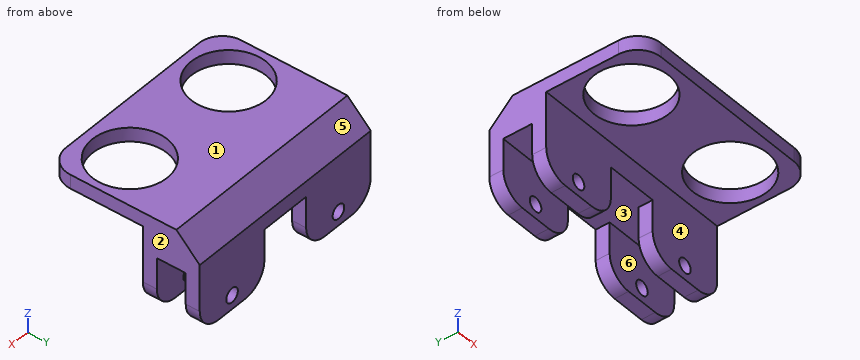
```python
from build123d import *

# Parameters (mm, degrees)
SKETCH1_R           = 8
BOSS_EXTRUDE1_DEPTH = 3
SKETCH2_W           = 17
SKETCH2_H           = 3
BOSS_EXTRUDE2_DEPTH = 17
SKETCH3_W           = 45
SKETCH3_H           = 3
BOSS_EXTRUDE3_DEPTH = 9.2
BOSS_EXTRUDE4_REACH = 41.571
SKETCH4_W           = 5.3
SKETCH4_H           = 3
SKETCH6_W           = 45
SKETCH6_H           = 5.3
BOSS_EXTRUDE5_DEPTH = 9.2
SKETCH7_W           = 17
SKETCH7_H           = 3
BOSS_EXTRUDE6_DEPTH = 11.7
SKETCH8_R           = 1.525
CUT_EXTRUDE1_DEPTH  = 44.180319591
CHAMFER1_SIZE       = 5
FILLET1_R           = 5


with BuildPart() as part:
    # Sketch1 → Boss-Extrude1 (new body)
    with BuildSketch(Plane.XY):
        with BuildLine():
            Line((-17.5, -10.5), (17.5, -10.5))
            ThreePointArc((17.5, -10.5), (21.035533906, -9.035533906), (22.5, -5.5))
            Line((22.5, -5.5), (22.5, 10.5))
            Line((22.5, 10.5), (22.5, 13))
            Line((22.5, 13), (-22.5, 13))
            Line((-22.5, 13), (-22.5, 10.5))
            Line((-22.5, 10.5), (-22.5, -5.5))
            ThreePointArc((-22.5, -5.5), (-21.035533906, -9.035533906), (-17.5, -10.5))
        make_face()
        with Locations((13, -0.5)):
            Circle(SKETCH1_R, mode=Mode.SUBTRACT)
        with Locations((-13, -0.5)):
            Circle(SKETCH1_R, mode=Mode.SUBTRACT)
    extrude(amount=BOSS_EXTRUDE1_DEPTH)

    # Sketch2 → Boss-Extrude2 (add)
    with BuildSketch(Plane(origin=(0, 0, 0), x_dir=(-1, 0, 0), z_dir=(0, 0, -1))):
        with Locations((-14, 11.5)):
            Rectangle(SKETCH2_W, SKETCH2_H)
        with Locations((14, 11.5)):
            Rectangle(SKETCH2_W, SKETCH2_H)
    extrude(amount=BOSS_EXTRUDE2_DEPTH)

    # Sketch3 → Boss-Extrude3 (add)
    with BuildSketch(Plane(origin=(0, 13, 0), x_dir=(1, 0, 0), z_dir=(0, 1, 0))):
        with Locations((0, -1.5)):
            Rectangle(SKETCH3_W, SKETCH3_H)
    extrude(amount=BOSS_EXTRUDE3_DEPTH)

    # Sketch4 → Boss-Extrude4 (add, up to next)
    with BuildSketch(Plane(origin=(-5.5, 0, 0), x_dir=(0, 0, -1), z_dir=(1, 0, 0)), mode=Mode.PRIVATE) as boss_extrude4_sk1:
        with Locations((2.65, 11.5)):
            Rectangle(SKETCH4_W, SKETCH4_H)
    boss_extrude4_tool1 = extrude(boss_extrude4_sk1.sketch, amount=BOSS_EXTRUDE4_REACH, mode=Mode.PRIVATE) - part.part
    add(boss_extrude4_tool1.solids().sort_by_distance((-5.5, 11.5, -2.65))[0])

    # Sketch6 → Boss-Extrude5 (add)
    with BuildSketch(Plane(origin=(0, 13, 0), x_dir=(1, 0, 0), z_dir=(0, 1, 0))):
        with Locations((0, 2.65)):
            Rectangle(SKETCH6_W, SKETCH6_H)
    extrude(amount=BOSS_EXTRUDE5_DEPTH)

    # Sketch7 → Boss-Extrude6 (add, through all)
    with BuildSketch(Plane(origin=(0, 0, -5.3), x_dir=(-1, 0, 0), z_dir=(0, 0, -1))):
        with Locations((-14, 20.7)):
            Rectangle(SKETCH7_W, SKETCH7_H)
        with Locations((14, 20.7)):
            Rectangle(SKETCH7_W, SKETCH7_H)
    extrude(amount=BOSS_EXTRUDE6_DEPTH)

    # Sketch8 → Cut-Extrude1 (cut, through all)
    with BuildSketch(Plane(origin=(0, 22.2, 0), x_dir=(1, 0, 0), z_dir=(0, 1, 0))):
        with Locations(Location((14, 14, 0), (0, 0, 270))):
            Circle(SKETCH8_R)
        with Locations(Location((-14, 14, 0), (0, 0, 270))):
            Circle(SKETCH8_R)
    extrude(amount=-CUT_EXTRUDE1_DEPTH, mode=Mode.SUBTRACT)

    # Chamfer1
    chamfer1_edges = [part.edges().sort_by_distance(p)[0] for p in [
        (0, 22.2, 3),
    ]]
    chamfer(chamfer1_edges, length=CHAMFER1_SIZE)

    # Fillet1
    fillet1_edges = [part.edges().sort_by_distance(p)[0] for p in [
        (22.5, 20.7, -17),
        (5.5, 20.7, -17),
        (-22.5, 20.7, -17),
        (-5.5, 20.7, -17),
        (5.5, 11.5, -17),
        (22.5, 11.5, -17),
        (-5.5, 11.5, -17),
        (-22.5, 11.5, -17),
    ]]
    fillet(fillet1_edges, radius=FILLET1_R)


solid = part.part
```
Geometry check sheet. Reference: the model listing, model coordinates, mm. Face numbers are marked on the shaded views. A direction names the side the tool comes from. Give positions to 0.01 mm unless a question says otherwise; leave off trailing zeros. Order: outer loops, then holes, each group sorted by start corner. A loop starts at its lowest first (then second) coordinate and runs counter-clockwise, first axis right, second up.
1. Thickness scan on L1, parallel to Y at x = 13, z = -6; L2, parallel to X at y = 11.65, z = -14 (3 decimals); L3, parallel to Z at x = -0.5, y = 10.5. Record the ranges inside material, lowest first.
2. Access from +Z, -Z, +X, -X, +Y, -Y to the whole of each face (thin tool, end or side, straight path). Record for the marked faces 4, 5 and 6.
3. Section check A-A, the plane y = -0.5. Enter the section's corners in (x, z), and give its area (3 significant figures).
4. Release check for a two-part mould opening along X. For the marked faces 1, 2 and 3 record: pulls with the +X half, pulls with the -X half, needs draft (parallel to the pull), parting line crosses it, or undercut.
5. Section check C-C, the plane y = 20. Enter the section's corners in (x, z) (3 decimals).
6. Gauge pin test, flat ends, axial feed: pin 1 Ø5 at (x, z) = (14, -14) entering from +Y; pin 2 Ø1.5 at (x, z) = (17.5, -14.5) entering from -Y; pin 3 Ø5 at (y, z) = (6, -15) entering from +X; pin 4 Ø2 at (x, y) = (-17.5, 18) entering from -Z. Record the tip position at first contact, or that the pin passes through.
7. Section check B-B, the plane z = -9. Enter the section's corners in (x, y), and give its area (3 significant figures).
8. Section check D-D, the plane x = -14. Enter the section's corners in (y, z) (3 decimals).
Values follow:
1. L1: y = 10 to 13, 19.2 to 22.2
1. L2: x = -22.083 to -15.525, -12.475 to -5.917, 5.917 to 12.475, 15.525 to 22.083
1. L3: z = -5.3 to 3
2. face 4: -Z, +X, -X, -Y
2. face 5: +Z, +X, -X, +Y
2. face 6: -Z, +X, -X
3. outline: (-22.5, 0) - (-21, 0) - (-21, 3) - (-22.5, 3) - close; (-5, 0) - (5, 0) - (5, 3) - (-5, 3) - close; (21, 0) - (22.5, 0) - (22.5, 3) - (21, 3) - close
3. area: 39.0 mm2
4. face 1: needs draft
4. face 2: pulls with the +X half
4. face 3: undercut
5. outline: (-22.5, -12) arc R5 ccw to (-17.5, -17) - (-10.5, -17) arc R5 ccw to (-5.5, -12) - (-5.5, -5.3) - (5.5, -5.3) - (5.5, -12) arc R5 ccw to (10.5, -17) - (17.5, -17) arc R5 ccw to (22.5, -12) - (22.5, 0.2) - (-22.5, 0.2) - close; hole circle Ø3.05 at (-14, -14); hole circle Ø3.05 at (14, -14)
6. pin 1: stops at y = 22.2
6. pin 2: stops at y = 10
6. pin 3: passes through
6. pin 4: stops at z = -5.3
7. outline: (-22.5, 10) - (-5.5, 10) - (-5.5, 13) - (-22.5, 13) - close; (-22.5, 19.2) - (-5.5, 19.2) - (-5.5, 22.2) - (-22.5, 22.2) - close; (5.5, 10) - (22.5, 10) - (22.5, 13) - (5.5, 13) - close; (5.5, 19.2) - (22.5, 19.2) - (22.5, 22.2) - (5.5, 22.2) - close
7. area: 204 mm2
8. outline: (-10.5, 0) - (-8.437, 0) - (-8.437, 3) - (-10.5, 3) - close; (7.437, 0) - (10, 0) - (10, -12.475) - (13, -12.475) - (13, -5.3) - (19.2, -5.3) - (19.2, -12.475) - (22.2, -12.475) - (22.2, -2) - (17.2, 3) - (7.437, 3) - close; (10, -17) - (13, -17) - (13, -15.525) - (10, -15.525) - close; (19.2, -17) - (22.2, -17) - (22.2, -15.525) - (19.2, -15.525) - close
